Autodesk Inventor part; units mm, degrees
ref_plane "YZ Plane" through (0, 0, 0) normal (1, 0, 0) x (0, 1, 0)
ref_plane "XZ Plane" through (0, 0, 0) normal (0, 1, 0) x (-1, 0, 0)
ref_plane "XY Plane" through (0, 0, 0) normal (0, 0, 1) x (1, 0, 0)
sketch "草图1" plane through (0, 0, 0) normal (0, 0, 1) x (1, 0, 0)
  line L0 (33, 0) -> (46.5, 0)
  line L1 (33, 5) -> (46.5, 5)
  line L2 (25, -72) -> (33, -72)
  line L3 (0, 0) -> (96, 0)
  line L4 (96, 0) -> (96, -72)
  line L5 (96, -72) -> (0, -72)
  line L6 (0, -72) -> (0, 0)
  line L7 (27, -69) -> (22, -69)
  line L8 (22, -69) -> (22, -10)
  line L9 (22, -10) -> (27, -10)
  line L10 (27, -10) -> (27, -69)
  line L11 (48, -81.8349) -> (48, 25.2825) construction
  line L12 (33, 0) -> (63, 0)
  line L13 (63, 0) -> (63, 5)
  line L14 (63, 5) -> (33, 5)
  line L15 (33, 5) -> (33, 0)
  line L16 (33, 0) -> (63, 5) construction
  line L17 (63, 0) -> (33, 5) construction
  line L18 (46, -77) -> (61, -77)
  line L19 (63, -72) -> (33, -72)
  line L20 (33, -72) -> (33, -77)
  line L21 (33, -77) -> (63, -77)
  line L22 (63, -77) -> (63, -72)
  circle A0 centre (48, 2.5) radius 1.5
  circle A1 centre (48, -74.5) radius 1.5
  line L23 (33, 5) -> (33, 0)
  line L24 (46.5, 0) -> (46.5, 5)
  dimension "d0" = 3
  dimension "d1" = 10
  dimension "d2" = 59
  dimension "d3" = 5
  dimension "d4" = 22
  dimension "d6" = 3
  dimension "d7" = 3
extrude "拉伸1" add sketch "草图1" along normal blind 5
properties part number "face"
The model under review builds one solid part; all positions refer to its coordinate system, in mm. A direction names the side the tool comes from. Coordinates: 2 decimals unless noted, no trailing zeros. Loops run counter-clockwise (first coordinate to the right, second up) from the corner with the lowest first, then second, coordinate; pieces in that order, holes last.
(1) Consider section D-D, the plane y = 2.5. Give the boundary of the cut face in (x, z), plus the area to 3 significant figures.
Determined:
outline: (33, 0) - (46.5, 0) - (46.5, 5) - (33, 5) - close; (49.5, 0) - (63, 0) - (63, 5) - (49.5, 5) - close
area: 135 mm2
(2) Tool access review of faces 5 (the flat face through (25, -69, 2)), 6 (the flat face through (79, 0, 2)), 7 (the flat face through (17, -72, 2)): name each direction out of +Z, -Z, +X, -X, +Y, -Y from which nothing blocks a thin tool from reaching the whole face with its end or side.
Determined:
face 5: +Z, -Z
face 6: +Z, -Z, +X, +Y
face 7: +Z, -Z, -X, -Y
(3) Wall thickness on L1, parallel to Y at x = 48, z = 2.2; L2, parallel to X at y = -20, z = 2.25; L3, parallel to X at y = -74.5, z = 1.15: over which ranges is each line inside the solid? List them lowest first.
Determined:
L1: y = -77 to -76, -73 to 1, 4 to 5
L2: x = 0 to 22, 27 to 96
L3: x = 33 to 46.5, 49.5 to 63
(4) Consider section C-C, the plane z = 3. Give the boundary of the cut face in (x, y), plus the area to 3 significant figures.
Determined:
outline: (0, -72) - (33, -72) - (33, -77) - (63, -77) - (63, -72) - (96, -72) - (96, 0) - (63, 0) - (63, 5) - (33, 5) - (33, 0) - (0, 0) - close; hole (22, -69) - (27, -69) - (27, -10) - (22, -10) - close; hole circle Ø3 at (48, -74.5); hole circle Ø3 at (48, 2.5)
area: 6,900 mm2
(5) Consider section A-A, the plane x = 48. Give the boundary of the cut face in (y, z).
Determined:
outline: (-77, 0) - (-76, 0) - (-76, 5) - (-77, 5) - close; (-73, 0) - (1, 0) - (1, 5) - (-73, 5) - close; (4, 0) - (5, 0) - (5, 5) - (4, 5) - close
(6) Insertion check: P1, Ø2, axis at x = 19.5, z = 1.5, coming from the +Y side; P2, Ø2.5, axis at y = 2, z = 3.5, coming from the +X side; P3, Ø1.5, axis at y = -75.5, z = 3, coming from the -X side. Each pin has a flat end and moves straight along its axis. Give the tip position at first contact, or say it passes through.
Determined:
P1: stops at y = 0
P2: stops at x = 63
P3: stops at x = 33
(7) Draft analysis for pull direction X (two halves, no side actions). For faces 1 (the flat face through (47, -35, 0)), 2 (the cylindrical face through (46.5, 2.43, 2.46)), 3 (the flat face through (63, -75, 2)), 4 (the flat face through (33, 3, 2)), state which applies: +X half, -X half, draft (parallel to the pull), parting line (faces both ways), or undercut.
Determined:
face 1: draft
face 2: undercut
face 3: +X half
face 4: -X half
(8) Consider section B-B, the plane y = -32.5. Give the boundary of the cut face in (x, z).
Determined:
outline: (0, 0) - (22, 0) - (22, 5) - (0, 5) - close; (27, 0) - (96, 0) - (96, 5) - (27, 5) - close
